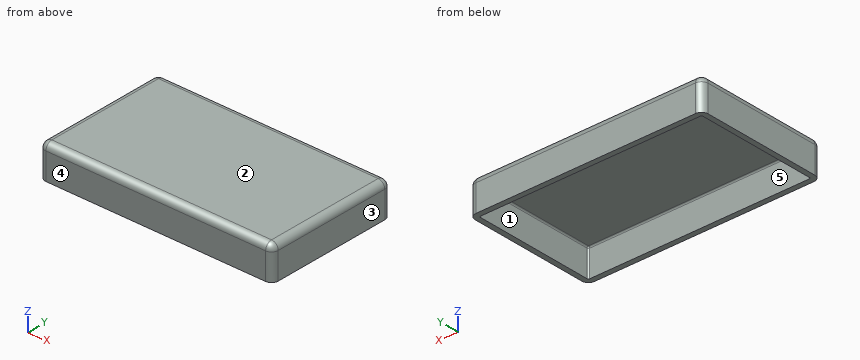
```python
from build123d import *

# Parameters (mm, degrees)
F0_W     = 88.9
F0_H     = 50.8
F1_DEPTH = 12.7
F2_R     = 2.54
F3_T     = -2


with BuildPart() as f1:
    # F0 (on Top) → F1 (new body)
    with BuildSketch(Plane.XY):
        Rectangle(F0_W, F0_H)
    extrude(amount=F1_DEPTH)

    # F2
    f2_edges = [f1.edges().sort_by_distance(p)[0] for p in [
        (0, -25.4, 12.7),
        (0, 25.4, 12.7),
        (44.45, 0, 12.7),
        (-44.45, 0, 12.7),
        (-44.45, 25.4, 6.35),
        (-44.45, -25.4, 6.35),
        (44.45, -25.4, 6.35),
        (44.45, 25.4, 6.35),
    ]]
    fillet(f2_edges, radius=F2_R)

    # F3
    f3_openings = [f1.faces().sort_by_distance(p)[0] for p in [
        (0, 0, 0),
    ]]
    offset(amount=F3_T, openings=f3_openings)


solid = f1.part
```
The listing builds one solid part. Answer for the finished solid, in the listing's coordinates (mm). Face numbers are marked on the shaded views. A direction names the side the tool comes from. Round coordinates to 2 decimals unless told otherwise and drop trailing zeros. Order: outer loops, then holes, each group sorted by start corner. A loop starts at its lowest first (then second) coordinate and runs counter-clockwise, first axis right, second up. Notation, with made-up numbers: (36.25, 88) - (40.25, 88) arc R23 ccw to (40.25, 122) - close; hole circle Ø5 at (35.5, -21.75). An arc over 180 degrees is marked (long way). Put each result on its own line as item: value. Start each with the question number.
(1) Given P1, Ø12, axis at x = -18.5, y = 5, coming from the -Z side, flat-ended and moving along its own axis, determine where the tip first touches the part or whether it passes through.
(2) Find section C-C (x = 5.5). Give the vertices of the cut face in (y, z).
(3) For the marked faces 4 and 5, determine the directions among +Z, -Z, +X, -X, +Y, -Y from which every point of the face is accessible in a straight line to the end or side of a thin tool.
(4) Straight lines are drawn through the part: probe 1 along X at (y, z) = (-13, 8.25); probe 2 along Y at (x, z) = (40, 10.25); probe 3 along Z at (x, y) = (5.5, -7). For each, find the intervals that lie inside material, in ascending order. Write a range as from..to.
(5) Find section A-A (z = 3.5). Give the vertices of the cut face in (x, y).
(6) Determine the mould class of the marked faces 1, 2 and 3 for opening direction X: released by +X, released by -X, zero draft, split by the parting line, or undercut.
(7) Find section B-B (y = -17). Give the vertices of the cut face in (x, z), plus the area to 3 significant figures.
Reply:
1. P1: z = 10.7
2. outline: (-25.4, 0) - (-23.4, 0) - (-23.4, 10.16) arc R0.54 cw to (-22.86, 10.7) - (22.86, 10.7) arc R0.54 cw to (23.4, 10.16) - (23.4, 0) - (25.4, 0) - (25.4, 10.16) arc R2.54 ccw to (22.86, 12.7) - (-22.86, 12.7) arc R2.54 ccw to (-25.4, 10.16) - close
3. face 4: +Z, -Z, +X, -X, -Y
3. face 5: -Z
4. probe 1: -44.45..-42.45, 42.45..44.45
4. probe 2: -25.4..-23.39, 23.39..25.4
4. probe 3: 10.7..12.7
5. outline: (-44.45, -22.86) arc R2.54 ccw to (-41.91, -25.4) - (41.91, -25.4) arc R2.54 ccw to (44.45, -22.86) - (44.45, 22.86) arc R2.54 ccw to (41.91, 25.4) - (-41.91, 25.4) arc R2.54 ccw to (-44.45, 22.86) - close; hole (-42.45, -22.86) arc R0.54 ccw to (-41.91, -23.4) - (41.91, -23.4) arc R0.54 ccw to (42.45, -22.86) - (42.45, 22.86) arc R0.54 ccw to (41.91, 23.4) - (-41.91, 23.4) arc R0.54 ccw to (-42.45, 22.86) - close
6. face 1: undercut
6. face 2: zero draft
6. face 3: released by +X
7. outline: (-44.45, 0) - (-42.45, 0) - (-42.45, 10.16) arc R0.54 cw to (-41.91, 10.7) - (41.91, 10.7) arc R0.54 cw to (42.45, 10.16) - (42.45, 0) - (44.45, 0) - (44.45, 10.16) arc R2.54 ccw to (41.91, 12.7) - (-41.91, 12.7) arc R2.54 ccw to (-44.45, 10.16) - close
7. area: 218 mm^2
